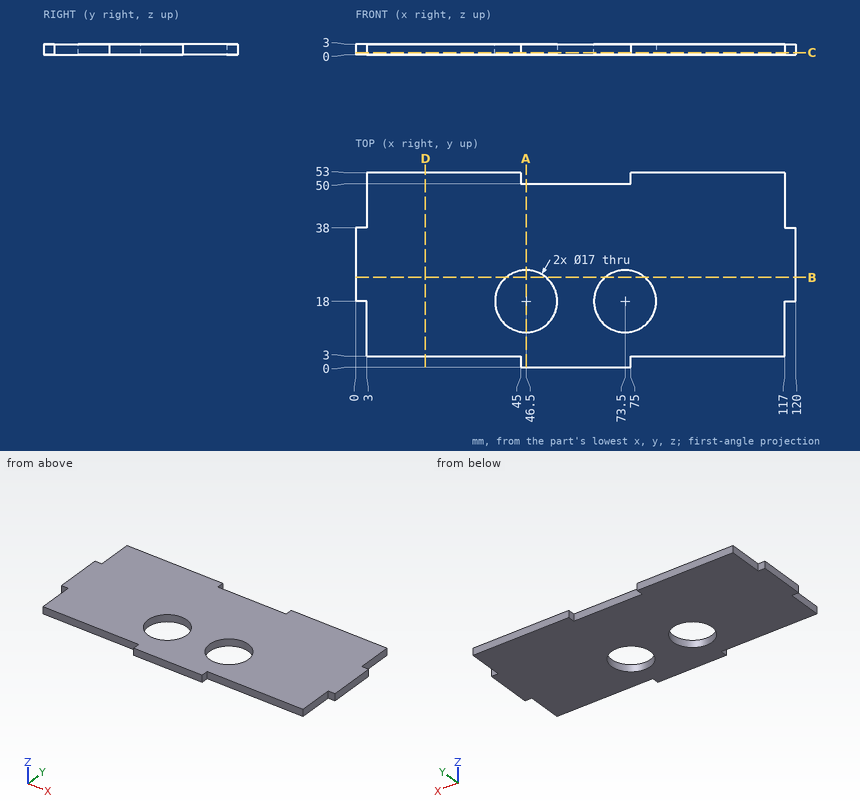
For this review, use the dimensioned drawing (mm, ordinates from the lowest corner) and the shaded views. Coordinates: 2 decimals unless noted, no trailing zeros. Order: outer loops, then holes, each group sorted by start corner. A loop starts at its lowest first (then second) coordinate and runs counter-clockwise, first axis right, second up. Notation, with made-up numbers: M 87.5,14.5 L 97.5,14.5 A20 cw 97.5,38.5 Z; hole C 66.5,-6 d7. An arc over 180 degrees is marked long. Answer as a JSON object with one key per item and string values. Group by question number.
1) Add section C-C, the plane z = 0.65. Write out the cut boundary in (x, y).
2) Wall thickness on L1, parallel to Y at x = 73.5, z = 0.95; L2, parallel to X at y = 15.5, z = 0.85; L3, parallel to X at y = 19.5, z = 1.9: over which ranges is each line inside the solid? List them lowest first.
3) Add section D-D, the plane x = 19. Write out the cut boundary in (y, z), then the cut area to 3 significant figures.
4) Add section A-A, the plane x = 46.5. Write out the cut boundary in (y, z).
5) Add section B-B, the plane y = 24.5. Write out the cut boundary in (x, z).
6) For pin 1 (8 mm diameter, centred on x = 52.5, y = 21.5, fed in from +Z); pin 2 (1.5 mm diameter, centred on y = 52, z = 1.5, fed in from +X); pin 3 (0.9 mm diameter, centred on x = 118, z = 2, fed in from +Y); pin 4 (1.5 mm diameter, centred on y = 47.5, z = 1, fed in from -X), all flat-tipped, find the tip position at first contact; note any pin that passes through.
Computed values:
{
 "1": {"outline": "M 0,18 L 3,18 L 3,3 L 45,3 L 45,0 L 75,0 L 75,3 L 117,3 L 117,18 L 120,18 L 120,38 L 117,38 L 117,53 L 75,53 L 75,50 L 45,50 L 45,53 L 3,53 L 3,38 L 0,38 Z; hole C 46.5,18 d17; hole C 73.5,18 d17"},
 "2": {"L1": "y = 0 to 9.5, 26.5 to 50", "L2": "x = 3 to 38.38, 54.62 to 65.38, 81.62 to 117", "L3": "x = 0 to 38.13, 54.87 to 65.13, 81.87 to 120"},
 "3": {"outline": "M 3,0 L 53,0 L 53,3 L 3,3 Z", "area": "150 mm^2"},
 "4": {"outline": "M 0,0 L 9.5,0 L 9.5,3 L 0,3 Z; M 26.5,0 L 50,0 L 50,3 L 26.5,3 Z"},
 "5": {"outline": "M 0,0 L 41.02,0 L 41.02,3 L 0,3 Z; M 51.98,0 L 68.02,0 L 68.02,3 L 51.98,3 Z; M 78.98,0 L 120,0 L 120,3 L 78.98,3 Z"},
 "6": {"pin 1": "stops at z = 3", "pin 2": "stops at x = 117", "pin 3": "stops at y = 38", "pin 4": "stops at x = 3"}
}
